Design review of the part built by this model. Coordinates are the model's own, in mm. Coordinates: 2 decimals unless noted, no trailing zeros. Loops run counter-clockwise (first coordinate to the right, second up) from the corner with the lowest first, then second, coordinate; pieces in that order, holes last. Notation, with made-up numbers: M 41.5,3 L 95.5,3 A21 ccw 95.5,18 Z; hole C 9,73.25 d4. An arc over 180 degrees is marked long. Put each result on its own line as item: value. Start each with the question number.
(1) Take a section at A-A, the plane z = -260. Give the boundary of the cut face in (x, y).
(2) Take a section at B-B, the plane x = -150. Give the boundary of the cut face in (y, z), then the cut area to 3 significant figures.
(3) For probe 1 along X at (y, z) = (2.25, -260); probe 2 along Z at (x, y) = (-150, 1.55); probe 3 along Z at (x, y) = (-156.5, 0.65), list the stretches that pass through material, from the lowest coordinate up. Write a range as [from, to].
Autodesk Inventor part; units mm, degrees
ref_plane "YZ Plane" through (0, 0, 0) normal (1, 0, 0) x (0, 1, 0)
ref_plane "XZ Plane" through (0, 0, 0) normal (0, 1, 0) x (-1, 0, 0)
ref_plane "XY Plane" through (0, 0, 0) normal (0, 0, 1) x (1, 0, 0)
sketch "Эскиз1" plane through (0, 0, 0) normal (0, 1, 0) x (-1, 0, 0)
  line L0 (0, 0) -> (200, 0)
  line L1 (200, 0) -> (200, -520)
  line L2 (200, -520) -> (0, -520)
  line L3 (0, -520) -> (0, 0)
  circle A0 centre (150, -260) radius 8
  line L4 (150, -260) -> (0, -260)
  line L5 (150, -260) -> (200, -260)
  dimension "d0" = 200
  dimension "d1" = 520
  dimension "d2" = 16
  dimension "d3" = 150
extrude "Выдавливание1" add sketch "Эскиз1" along normal blind 4 contours L0 L1 L5 A0 L4 L3 | L4 A0 L5 L1 L2 L3
properties part number "Стена 16 мм отверстие"
Computed values:
1. outline: M -200,0 L -158,0 L -158,4 L -200,4 Z; M -142,0 L 0,0 L 0,4 L -142,4 Z
2. outline: M 0,-520 L 4,-520 L 4,-268 L 0,-268 Z; M 0,-252 L 4,-252 L 4,0 L 0,0 Z
2. area: 2,020 mm^2
3. probe 1: x = [-200, -158], [-142, 0]
3. probe 2: z = [-520, -268], [-252, 0]
3. probe 3: z = [-520, -264.66], [-255.34, 0]
